from build123d import *

# Parameters (mm, degrees)
F0_R     = 1
F1_DEPTH = 3
F5_START = -42
F5_DEPTH = 9


with BuildPart() as f1:
    # F0 (on Front) → F1 (new body)
    with BuildSketch(Plane.XZ):
        Polygon((-52.5, -46), (52.5, -46), (46.5, 34), (30, 46), (-30, 46), (-46.5, 34), align=None)
        with Locations((-7, -4.2)):
            Circle(F0_R, mode=Mode.SUBTRACT)
        with BuildLine():
            ThreePointArc((8, -4.2), (7, -5.2), (6, -4.2))
            ThreePointArc((6, -4.2), (7, -3.2), (8, -4.2))
        make_face(mode=Mode.SUBTRACT)
    extrude(amount=-F1_DEPTH)

    # F2 (on Top) → F3 (revolve)
    with BuildSketch(Plane.XY):
        Polygon((-28, 0), (-1.999999598, 50.0012680348), (-4.9999989951, 50.0031700871), (-12, 36.5407767282), (-31, 0), align=None)
        Polygon((-12, 36.5407767282), (-4.9999989951, 50.0031700871), (-12, 50.0076082106), align=None)
    revolve(axis=Axis((0, 25, 0), (0, 1, 0)))

    # F2 (on Top) → F4 (revolve, cut)
    with BuildSketch(Plane.XY):
        Polygon((-20, 0), (-2, 0), (-1.999999598, 50.0012680348), (-28, 0), (-22, 0), align=None)
        Polygon((-2, 0), (0, 0), (0, 50), (-1.999999598, 50.0012680348), align=None)
    revolve(axis=Axis((0, 50.0012680348, 0), (0, 1, 0)), mode=Mode.SUBTRACT)

    # F0 (on Front) → F5 (cut)
    with BuildSketch(Plane.XZ.offset(F5_START)):
        with BuildLine():
            ThreePointArc((8, -4.2), (7, -3.2), (6, -4.2))
            ThreePointArc((6, -4.2), (7, -5.2), (8, -4.2))
        make_face()
        with Locations((-7, -4.2)):
            Circle(F0_R)
    extrude(amount=-F5_DEPTH, mode=Mode.SUBTRACT)


solid = f1.part
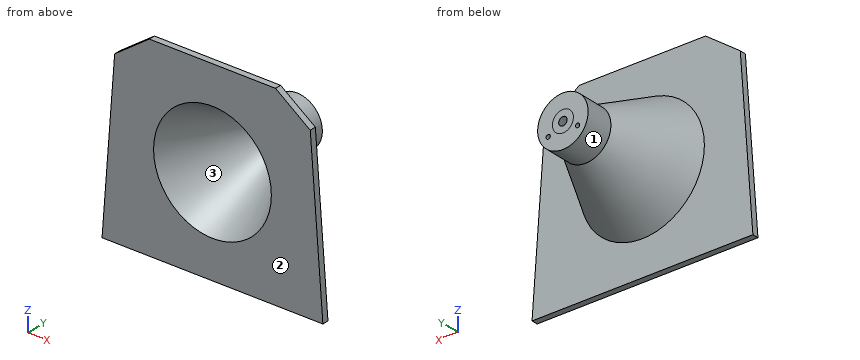
The listing builds one solid part. Answer for the finished solid, in the listing's coordinates (mm). Face numbers are marked on the shaded views. Round coordinates to 2 decimals unless told otherwise and drop trailing zeros. Write each loop counter-clockwise with the first axis right and the second up, starting at its lowest first coordinate (ties: lowest second). Pieces come first, ordered by that corner, then holes. Notation, with made-up numbers: (46.5, 1.5) - (98.5, 1.5) arc R8 cw to (98.5, 14.5) - close; hole circle Ø3 at (68, 17). An arc over 180 degrees is marked (long way). Use one line per item in the form item = value. Start each with the question number.
Item 1: Determine the mould class of the marked faces 1, 2 and 3 for opening direction X: +X half, -X half, draft (parallel to the pull), parting line (faces both ways), or undercut.
Item 2: Flat-ended cylindrical pins translate along their axes: pin 1 Ø1.5 at (x, y) = (-11, 35.5) entering from +Z; pin 2 Ø8 at (x, y) = (-1, 32) entering from +Z; pin 3 Ø5 at (x, z) = (-28.5, -26) entering from -Y; pin 4 Ø1 at (x, z) = (6.5, -4) entering from +Y. Find the tip coordinate at first contact, or state that the pin passes through.
Item 3: Find the intervals of material crossed by line 1 (Y direction, x = -43, z = 17.5); line 2 (X direction, y = 44, z = -4); line 3 (Z direction, x = -7, y = 46.5), in increasing order. Write a range as [from, to].
Item 4: A cutting plane is placed at B-B (y = 7). Write down the section's boundary in (x, z), plus the area to 3 significant figures.
Item 5: A cutting plane is placed at A-A (y = 35). Write down the section's boundary in (x, z).
The answers:
q1.face_1 = parting line
q1.face_2 = draft
q1.face_3 = undercut
q2.pin_1 = 7.42
q2.pin_2 = 16.42
q2.pin_3 = 0
q2.pin_4 = 50
q3.line_1 = [0, 3]
q3.line_2 = [-11.31, -7.98], [-6.02, -3.2], [3.2, 6.02], [7.98, 11.31]
q3.line_3 = [-9.75, -5.2], [-3.2, 9.75]
q4.outline = circle Ø54.72 at (0, 0); hole circle Ø48.72 at (0, 0)
q4.area = 487 mm^2
q5.outline = circle Ø25.6 at (0, 0); hole circle Ø19.6 at (0, 0)
